Check sheet for the modelled part. Datum: model origin and axes. Units: mm. A direction names the side the tool comes from. Round coordinates to 2 decimals unless told otherwise and drop trailing zeros. Order: outer loops, then holes, each group sorted by start corner. A loop starts at its lowest first (then second) coordinate and runs counter-clockwise, first axis right, second up.
(1) Mould release check, pull along X, two halves, no side actions. Record for faces 4 (the cylindrical face through (0, -8, -3)), 5 (the flat face through (0, 10, 0)), 6 (the flat face through (2.2, 17.5, -2.2)): released by +X, released by -X, zero draft, split by the parting line, or undercut.
(2) Thickness scan on probe 1 along Z at (x, y) = (0, 0); probe 2 along Y at (x, z) = (0.25, -1.5). Record the ranges inside material, lowest first.
(3) Sectioned sample at D-D, the plane y = 20.5. Enter the section's corners in (x, z), and give its area (3 significant figures).
(4) Depth check by flat-ended pin: pin 1 (1.5 mm diameter, centred on x = 2, z = 1, fed in from +Y); pin 2 (1.5 mm diameter, centred on x = -2, y = -9, fed in from -Z); pin 3 (1 mm diameter, centred on x = -0.5, z = 0.5, fed in from -Y); pin 4 (1.5 mm diameter, centred on y = -4.5, z = -1.5, fed in from +X). Enter the tip coordinate at first touch or a pass-through.
(5) Sectioned sample at C-C, the plane y = 4.5. Enter the section's corners in (x, z), and give its area (3 significant figures).
(6) Tool access check on faces 1 (the cylindrical face through (2.685, 21.05, -0.596)), 2 (the flat face through (1.3, -15, 1.3)), 3 (the cylindrical face through (0.97, -2.33, -1.27)). Record the directions out of +Z, -Z, +X, -X, +Y, -Y that give a thin tool (end or side, any length) a straight path to the whole face; none if there is none.
```python
from build123d import *

# Parameters (mm, degrees)
FILLET1_R      = 1
CHAMFER1_SIZE  = 15
CHAMFER1_SIZE2 = 1.974787464


with BuildPart() as part:
    # Sketch1 → Revolve1 (revolve)
    with BuildSketch(Plane(origin=(0, 0, 0), x_dir=(0, 0, -1), z_dir=(1, 0, 0))):
        Polygon((-2.75, 25.7), (-2.75, 17.5), (-5, 17.5), (-5, 15), (-3, 15), (-3, -15), (-1.6, -15), (-1.6, 10), (0, 10), (0, 25.7), align=None)
    revolve(axis=Axis((0, 26.571382603, 0), (0, -1, 0)))

    # Fillet1
    fillet1_edges = [part.edges().sort_by_distance(p)[0] for p in [
        (0, 25.7, -2.75),
    ]]
    fillet(fillet1_edges, radius=FILLET1_R)

    # Chamfer1
    chamfer1_edges = [part.edges().sort_by_distance(p)[0] for p in [
        (0, 15, -3),
    ]]
    chamfer1_side = [part.faces().sort_by_distance(p)[0] for p in [
        (0, 0, -3),
    ]]
    chamfer(chamfer1_edges, length=CHAMFER1_SIZE, length2=CHAMFER1_SIZE2, reference=chamfer1_side[0])


solid = part.part
```
Derived:
1. face 4: split by the parting line
1. face 5: undercut
1. face 6: zero draft
2. probe 1: z = -3 to -1.6, 1.6 to 3
2. probe 2: y = 10 to 25.7
3. outline: circle Ø5.5 at (0, 0)
3. area: 23.8 mm2
4. pin 1: stops at y = 25.7
4. pin 2: stops at z = -2.73
4. pin 3: stops at y = 10
4. pin 4: stops at x = 2.9
5. outline: circle Ø7.18 at (0, 0); hole circle Ø3.2 at (0, 0)
5. area: 32.5 mm2
6. face 1: +Y
6. face 2: +Z, -Z, +X, -X, -Y
6. face 3: -Y
